The model under review builds one solid part; all positions refer to its coordinate system, in mm. Face numbers are marked on the shaded views. A direction names the side the tool comes from. Round coordinates to 2 decimals unless told otherwise and drop trailing zeros. Order: outer loops, then holes, each group sorted by start corner. A loop starts at its lowest first (then second) coordinate and runs counter-clockwise, first axis right, second up. Notation, with made-up numbers: M 63.5,41.25 L 84.5,41.25 A19 ccw 84.5,62.25 Z; hole C 16,85 d10. An arc over 180 degrees is marked long. Answer as a JSON object with one key per item and string values. Group by question number.
1. Add section C-C on x = -6. State the section outline as (y, z) points, and give its area (3 significant figures).
2. To check wall thickness, follow probe 1 along Y at (x, z) = (5.25, 9); probe 2 along X at (y, z) = (1.5, 12.5) (3 decimals); probe 3 along Y at (x, z) = (26.5, 9.5). State the ranges of each line that lie inside material, in increasing order. Write a range as [from, to].
3. Machinability: for the marked faces 1, 2 and 3, which of the approach directions +Z, -Z, +X, -X, +Y, -Y give a long, thin tool a straight path to every point of the face, cutting with its end or side? Answer none if there is none.
4. Mouldability with a two-part tool opening along Y and no side actions: class the marked faces 4, 5 and 6 as released by +Y, released by -Y, zero draft, split by the parting line, or undercut.
5. Add section A-A on x = 76.7. State the section outline as (y, z) points, and give its area (3 significant figures).
6. Clearance check with flat-ended pins moving along their axes: P1, Ø9, axis at y = 56, z = 11.5, coming from the -X side; P2, Ø9, axis at y = -11, z = 10, coming from the +X side; P3, Ø1, axis at y = 19.5, z = 6, coming from the +X side. State where each tip first meets the part, or that it passes through.
7. Add section D-D on z = 9. Give the number of separate pieces and of enclosed holes in the cut face, and give its area (3 significant figures).
8. Add section B-B on y = -4.5. State the section outline as (x, z) points, and give its area (3 significant figures).
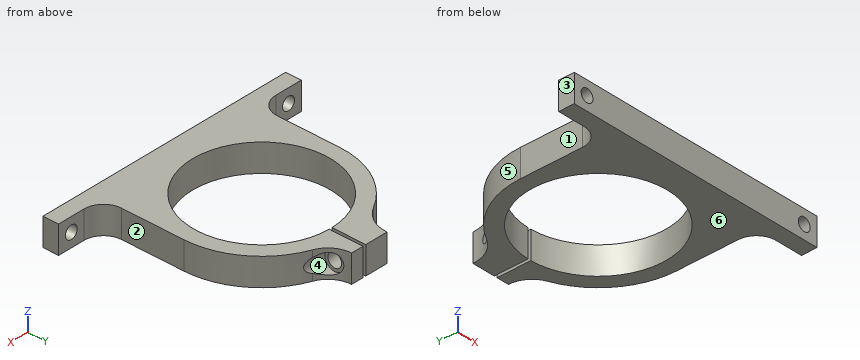
```python
from build123d import *

# Parameters (mm, degrees)
MAIN_BODY_DEPTH               = 18
SKETCH10_R                    = 6.5
HEAD_COUNTERBORE_DEPTH        = 18
TO_TABLE_M8_CLEARANCE_HOLE1_D = 8.4
SKETCH19_W                    = 3.4
SKETCH19_H                    = 84.7
M8_CLEARANCE_HOLE2_REACH      = 119.393
M8_CLEARANCE_HOLE2_BORE_R     = 4.5


with BuildPart() as part:
    # Sketch1 → main body (new body)
    with BuildSketch(Plane.XY):
        with BuildLine():
            Line((85.7, -53.34), (85.7, -63.5))
            Line((85.7, -63.5), (-85.7, -63.5))
            Line((-85.7, -63.5), (-85.7, -53.34))
            Line((-85.7, -53.34), (-67.7, -53.34))
            ThreePointArc((-67.7, -53.34), (-58.719743879, -49.620256121), (-55, -40.64))
            Line((-55, -40.64), (-55, 0))
            ThreePointArc((-55, 0), (-47.533550635, 27.668783205), (-27.161397671, 47.825291181))
            ThreePointArc((-27.161397671, 47.825291181), (-18.99354147, 55.906688319), (-16, 67))
            Line((-16, 67), (-1, 67))
            Line((-1, 67), (-1, 44.988887517))
            ThreePointArc((-1, 44.988887517), (0, -45), (1, 44.988887517))
            Line((1, 44.988887517), (1, 67))
            Line((1, 67), (9, 67))
            ThreePointArc((9, 67), (11.948921757, 57.494782102), (19.76003028, 51.327781983))
            ThreePointArc((19.76003028, 51.327781983), (45.342042661, 31.130357648), (55, 0))
            Line((55, 0), (55, -40.64))
            ThreePointArc((55, -40.64), (58.719743879, -49.620256121), (67.7, -53.34))
            Line((67.7, -53.34), (85.7, -53.34))
        make_face()
    extrude(amount=MAIN_BODY_DEPTH)

    # Sketch10 → head counterbore (cut)
    with BuildSketch(Plane.ZY.offset(-9)):
        with Locations((9, 55.994443758)):
            Circle(SKETCH10_R)
    extrude(amount=-HEAD_COUNTERBORE_DEPTH, mode=Mode.SUBTRACT)

    # to table M8 Clearance Hole1 (through all)
    with Locations(Plane(origin=(0, -53.34, 0), x_dir=(1, 0, 0), z_dir=(0, 1, 0))):
        with Locations((-76.7, -9), (76.7, -9)):
            Hole(TO_TABLE_M8_CLEARANCE_HOLE1_D / 2)

    # Sketch19 → M8x1.25 Tapped Hole1 (revolve, cut)
    with BuildSketch(Plane(origin=(-1, 55.994443758, 9), x_dir=(0, 0, -1), z_dir=(0, 1, 0))):
        with Locations((1.7, 42.35)):
            Rectangle(SKETCH19_W, SKETCH19_H)
    revolve(axis=Axis((5.35, 55.994443758, 9), (-1, 0, 0)), mode=Mode.SUBTRACT)

    # M8 Clearance Hole2 bore → M8 Clearance Hole2 (cut, up to next)
    with BuildSketch(Plane(origin=(9, 0, 0), x_dir=(0, 0, 1), z_dir=(1, 0, 0)), mode=Mode.PRIVATE) as m8_clearance_hole2_sk1:
        with Locations((9, -55.994443758)):
            Circle(M8_CLEARANCE_HOLE2_BORE_R)
    m8_clearance_hole2_tool1 = extrude(m8_clearance_hole2_sk1.sketch, amount=-M8_CLEARANCE_HOLE2_REACH, mode=Mode.PRIVATE) & part.part
    add(m8_clearance_hole2_tool1.solids().sort_by_distance((9, 55.994444, 9))[0], mode=Mode.SUBTRACT)


solid = part.part
```
Recorded:
{
 "1": {"outline": "M -63.5,0 L -44.6,0 L -44.6,18 L -63.5,18 Z; M 44.6,0 L 67,0 L 67,18 L 44.6,18 Z; hole C 55.99,9 d6.8", "area": "707 mm²"},
 "2": {"probe 1": "y = [-63.5, -44.69], [44.69, 51.49], [60.49, 67]", "probe 2": "x = [-54.98, -44.975], [44.975, 54.98]", "probe 3": "y = [-63.5, -36.37], [36.37, 48.19]"},
 "3": {"face 1": "+Z, -Z, -X, +Y", "face 2": "+Z, -Z, +X, +Y", "face 3": "+Z, -Z, -X, +Y, -Y"},
 "4": {"face 4": "undercut", "face 5": "released by +Y", "face 6": "zero draft"},
 "5": {"outline": "M -63.5,0 L -53.34,0 L -53.34,4.8 L -63.5,4.8 Z; M -63.5,13.2 L -53.34,13.2 L -53.34,18 L -63.5,18 Z", "area": "97.5 mm²"},
 "6": {"P1": "stops at x = -22.37", "P2": "stops at x = 55", "P3": "stops at x = 51.61"},
 "7": {"separate pieces": "5", "enclosed holes": "0", "area": "5,970 mm²"},
 "8": {"outline": "M -55,0 L -44.77,0 L -44.77,18 L -55,18 Z; M 44.77,0 L 55,0 L 55,18 L 44.77,18 Z", "area": "368 mm²"}
}
